Design review of the part built by this model. Coordinates are the model's own, in mm. A direction names the side the tool comes from. Round coordinates to 2 decimals unless told otherwise and drop trailing zeros. Order: outer loops, then holes, each group sorted by start corner. A loop starts at its lowest first (then second) coordinate and runs counter-clockwise, first axis right, second up. Notation, with made-up numbers: (-21, 36) - (6, 36) arc R28 ccw to (6, 57) - close; hole circle Ø7 at (-5.75, 78). An arc over 180 degrees is marked (long way). Use CSV: the item, a comma, the result in double quotes.
from build123d import *

# Parameters (mm, degrees)
SKETCH2_W           = 130
SKETCH2_H           = 120
BOSS_EXTRUDE1_DEPTH = 5
SKETCH3_W           = 126
SKETCH3_H           = 4
BOSS_EXTRUDE2_DEPTH = 52
SKETCH5_R           = 35
CUT_EXTRUDE1_DEPTH  = 2
SKETCH7_W           = 10
SKETCH7_H           = 10
BOSS_EXTRUDE3_DEPTH = 20
SKETCH9_W           = 4
SKETCH9_H           = 52
CUT_EXTRUDE2_DEPTH  = 5


with BuildPart() as part:
    # Sketch2 → Boss-Extrude1 (new body)
    with BuildSketch(Plane(origin=(0, 0, 0), x_dir=(1, 0, 0), z_dir=(0, 1, 0))):
        Rectangle(SKETCH2_W, SKETCH2_H)
    extrude(amount=BOSS_EXTRUDE1_DEPTH)

    # Sketch3 → Boss-Extrude2 (add)
    with BuildSketch(Plane.XZ):
        with Locations((-2, 58)):
            Rectangle(SKETCH3_W, SKETCH3_H)
    extrude(amount=BOSS_EXTRUDE2_DEPTH)

    # Sketch5 → Cut-Extrude1 (cut)
    with BuildSketch(Plane(origin=(0, 5, 0), x_dir=(1, 0, 0), z_dir=(0, 1, 0))):
        with Locations(Location((15, 5, 0), (0, 0, 270))):
            Circle(SKETCH5_R)
    extrude(amount=-CUT_EXTRUDE1_DEPTH, mode=Mode.SUBTRACT)

    # Sketch7 → Boss-Extrude3 (add)
    with BuildSketch(Plane.XZ):
        with Locations((-56, 40.5)):
            Rectangle(SKETCH7_W, SKETCH7_H)
        with Locations((56, 40.5)):
            Rectangle(SKETCH7_W, SKETCH7_H)
    extrude(amount=BOSS_EXTRUDE3_DEPTH)

    # Sketch9 → Cut-Extrude2 (cut)
    with BuildSketch(Plane(origin=(0, 0, 56), x_dir=(-1, 0, 0), z_dir=(0, 0, -1))):
        with Locations((63, -26)):
            Rectangle(SKETCH9_W, SKETCH9_H)
    extrude(amount=-CUT_EXTRUDE2_DEPTH, mode=Mode.SUBTRACT)


solid = part.part
1) We need section D-D (z = -5). Give the boundary of the cut face in (x, y), then the cut area to 3 significant figures.
Data:
outline,"(-65, 0) - (65, 0) - (65, 5) - (50, 5) - (50, 3) - (-20, 3) - (-20, 5) - (-65, 5) - close"
area,"510 mm2"
2) For faces 1 (the face through (-6, 4, -33)), 2 (the face through (56, -20, 41)), 3 (the face through (-61, -26, 58)), list the 3-axis set-ups (+Z, -Z, +X, -X, +Y, -Y) from which the entire face can be reached by the end or side of a thin tool; tool diameter is ignored.
Data:
face 1,"+Y"
face 2,"-Z, +X, -X, -Y"
face 3,"+Z, -Z, -X, -Y"
3) We need section C-C (y = -34.5). Give the boundary of the cut face in (x, z), then the cut area to 3 significant figures.
Data:
outline,"(-61, 56) - (61, 56) - (61, 60) - (-61, 60) - close"
area,"488 mm2"
4) The part is to be moulded in two halves that separate along Z. For faces 4 (the face through (-1, -23, 60)), 5 (the face through (61, -26, 58)), 6 (the face through (15, 3, -5)), say which applies: +Z half, -Z half, draft (parallel to the pull), parting line (faces both ways), or undercut.
Data:
face 4,"+Z half"
face 5,"draft"
face 6,"undercut"
5) To check wall thickness, follow L1, parallel to X at y = 4.3, z = -5; L2, parallel to Z at x = 16, y = -32.5; L3, parallel to Y at x = -59, z = -19. State the ranges of each line that lie inside material, in increasing order. Write a range as from..to.
Data:
L1,"x = -65..-20, 50..65"
L2,"z = 56..60"
L3,"y = 0..5"
6) We need section A-A (x = 15). Give the boundary of the cut face in (y, z), then the cut area to 3 significant figures.
Data:
outline,"(-52, 56) - (0, 56) - (0, -60) - (5, -60) - (5, -40) - (3, -40) - (3, 30) - (5, 30) - (5, 60) - (-52, 60) - close"
area,"668 mm2"
7) We need section B-B (z = 39). Give the boundary of the cut face in (x, y).
Data:
outline,"(-65, 0) - (-61, 0) - (-61, -20) - (-51, -20) - (-51, 0) - (51, 0) - (51, -20) - (61, -20) - (61, 0) - (65, 0) - (65, 5) - (-65, 5) - close"
8) Insertion check: pin 1 Ø1.5 at (x, z) = (-18.5, -6) entering from -Y; pin 2 Ø8 at (x, z) = (57, 38.5) entering from -Y; pin 3 Ø15.5 at (x, y) = (8, -27) entering from -Z. Each pin has a flat end and moves straight along its axis. Give the tip position at first contact, or say it passes through.
Data:
pin 1,"stops at y = 0"
pin 2,"stops at y = -20"
pin 3,"stops at z = 56"
